from build123d import *

# Parameters (mm, degrees)
SKETCH1_R           = 1.6
SKETCH1_R_2         = 8
SKETCH1_R_3         = 2.5
BOSS_EXTRUDE2_DEPTH = 6.35
CHAMFER2_SIZE       = 5
FILLET1_R           = 3
FILLET2_R           = 5


with BuildPart() as part:
    # Sketch1 → Boss-Extrude2 (new body)
    with BuildSketch(Plane(origin=(0, 0, 0), x_dir=(1, 0, 0), z_dir=(0, 1, 0))):
        Polygon((-21.15, 21.15), (21.15, 21.15), (21.15, 7.5), (95, 7.5), (95, -7.5), (21.15, -7.5), (21.15, -21.15), (-21.15, -21.15), align=None)
        with Locations(Location((-15.5, 15.5, 0), (0, 0, 270))):
            Circle(SKETCH1_R, mode=Mode.SUBTRACT)
        with Locations(Location((15.5, 15.5, 0), (0, 0, 270))):
            Circle(SKETCH1_R, mode=Mode.SUBTRACT)
        with Locations(Location((15.5, -15.5, 0), (0, 0, 270))):
            Circle(SKETCH1_R, mode=Mode.SUBTRACT)
        with Locations(Location((-15.5, -15.5, 0), (0, 0, 270))):
            Circle(SKETCH1_R, mode=Mode.SUBTRACT)
        with Locations(Location((0, 0, 0), (0, 0, 270))):
            Circle(SKETCH1_R_2, mode=Mode.SUBTRACT)
        with Locations(Location((90, 0, 0), (0, 0, 270))):
            Circle(SKETCH1_R_3, mode=Mode.SUBTRACT)
        with Locations(Location((55, 0, 0), (0, 0, 270))):
            Circle(SKETCH1_R_3, mode=Mode.SUBTRACT)
    extrude(amount=BOSS_EXTRUDE2_DEPTH)

    # Chamfer2
    chamfer2_edges = [part.edges().sort_by_distance(p)[0] for p in [
        (21.15, 3.175, 21.15),
        (-21.15, 3.175, 21.15),
        (-21.15, 3.175, -21.15),
        (21.15, 3.175, -21.15),
    ]]
    chamfer(chamfer2_edges, length=CHAMFER2_SIZE)

    # Fillet1
    fillet1_edges = [part.edges().sort_by_distance(p)[0] for p in [
        (95, 3.175, -7.5),
        (95, 3.175, 7.5),
    ]]
    fillet(fillet1_edges, radius=FILLET1_R)

    # Fillet2
    fillet2_edges = [part.edges().sort_by_distance(p)[0] for p in [
        (21.15, 3.175, -7.5),
        (21.15, 3.175, 7.5),
    ]]
    fillet(fillet2_edges, radius=FILLET2_R)


solid = part.part
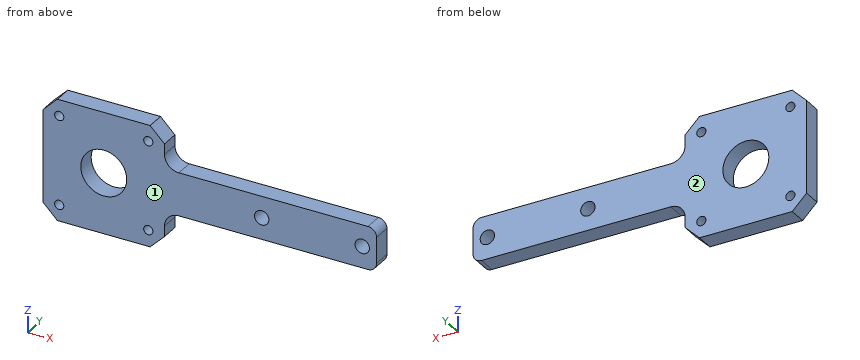
Source: CAD feature listing. Evaluate the final solid. Frame: model axes, mm. Face numbers are marked on the shaded views. Coordinates: 2 decimals unless noted, no trailing zeros. Order: outer loops, then holes, each group sorted by start corner. A loop starts at its lowest first (then second) coordinate and runs counter-clockwise, first axis right, second up. Notation, with made-up numbers: M 41.5,62 L 87.5,62 A19 cw 87.5,70 Z; hole C 42.25,-8 d9. An arc over 180 degrees is marked long. Write each question's results on one line, items separated by ' | '. Start each with the question number.
1. Section A-A, the plane y = 5. Return the cut outline in (x, z), then the cut area to 3 significant figures.
2. Section D-D, the plane z = -15. Return the cut outline in (x, y).
3. Section B-B, the plane x = 0. Return the cut outline in (y, z), then the cut area to 3 significant figures.
4. Section C-C, the plane z = 0. Return the cut outline in (x, y).
5. Material intervals for L1, parallel to X at y = 1, z = 0; L2, parallel to X at y = 4.25, z = 15.5; L3, parallel to Z at x = 43, y = 3.5, sorted ascending.
6. Pin query (flat end, axial travel): pin 1 (9.5 mm diameter, centred on x = 0, z = 0, fed in from +Y); pin 2 (1.1 mm diameter, centred on y = 3.5, z = 14.5, fed in from +X); pin 3 (1.9 mm diameter, centred on x = 57.5, y = 4, fed in from -Z); pin 4 (3 mm diameter, centred on x = 53, y = 2, fed in from +Z). Return the tip coordinate at first contact, or that it passes through.
7. Draft query along Y for the marked faces 1 and 2. Return one class per face: +Y half, -Y half, draft (parallel to the pull), parting line (faces both ways), or undercut.
Solution:
1) outline: M -21.15,-16.15 L -16.15,-21.15 L 16.15,-21.15 L 21.15,-16.15 L 21.15,-12.5 A5 cw 26.15,-7.5 L 92,-7.5 A3 ccw 95,-4.5 L 95,4.5 A3 ccw 92,7.5 L 26.15,7.5 A5 cw 21.15,12.5 L 21.15,16.15 L 16.15,21.15 L -16.15,21.15 L -21.15,16.15 Z; hole C -15.5,-15.5 d3.2; hole C -15.5,15.5 d3.2; hole C 0,0 d16; hole C 15.5,-15.5 d3.2; hole C 15.5,15.5 d3.2; hole C 55,0 d5; hole C 90,0 d5 | area: 2,580 mm²
2) outline: M -21.15,0 L -17.02,0 L -17.02,6.35 L -21.15,6.35 Z; M -13.98,0 L 13.98,0 L 13.98,6.35 L -13.98,6.35 Z; M 17.02,0 L 21.15,0 L 21.15,6.35 L 17.02,6.35 Z
3) outline: M 0,-21.15 L 6.35,-21.15 L 6.35,-8 L 0,-8 Z; M 0,8 L 6.35,8 L 6.35,21.15 L 0,21.15 Z | area: 167 mm²
4) outline: M -21.15,0 L -8,0 L -8,6.35 L -21.15,6.35 Z; M 8,0 L 52.5,0 L 52.5,6.35 L 8,6.35 Z; M 57.5,0 L 87.5,0 L 87.5,6.35 L 57.5,6.35 Z; M 92.5,0 L 95,0 L 95,6.35 L 92.5,6.35 Z
5) L1: -21.15 to -8, 8 to 52.5, 57.5 to 87.5, 92.5 to 95 | L2: -21.15 to -17.1, -13.9 to 13.9, 17.1 to 21.15 | L3: -7.5 to 7.5
6) pin 1: through | pin 2: x = 21.15 | pin 3: z = -7.5 | pin 4: z = 7.5
7) face 1: -Y half | face 2: +Y half
